```python
from build123d import *

# Parameters (mm, degrees)
CUT_EXTRUDE_1_DEPTH      = 43.811678643
PATTERN_CIRCULAR_5_COUNT = 3
EXTRUDE_1_DEPTH          = 4
SKETCH_5_R               = 14
CUT_EXTRUDE_2_DEPTH      = 45.179631373
SKETCH_6_R               = 7
CUT_EXTRUDE_3_DEPTH      = 45.17963138
SKETCH_7_W               = 30.2
SKETCH_7_H               = 16.2
CUT_EXTRUDE_4_DEPTH      = 3.35
EXTRUDE_START            = -0.2
SKETCH_8_R               = 7
EXTRUDE_2_DEPTH          = 0.2


with BuildPart() as part:
    # Sketch 1 → Revolve 1 (revolve)
    with BuildSketch(Plane.XY):
        with BuildLine():
            Line((11.135528726, 0), (28.991378029, 0))
            Line((28.991378029, 0), (28.991378029, 10.908116908))
            Line((28.991378029, 10.908116908), (27.577164466, 12.32233047))
            Line((27.577164466, 12.32233047), (26.673957337, 12.32233047))
            ThreePointArc((26.673957337, 12.32233047), (19.883391716, 4.927091635), (11.135528726, 0))
        make_face()
    revolve(axis=Axis((0, 0, 0), (0, 1, 0)))

    # Sketch 2 → Cut-Extrude 1 (cut, through all)
    with BuildSketch(Plane.XZ):
        with BuildLine():
            Line((4.04141358, 7), (4.04141358, -7))
            Line((4.04141358, -7), (34.14370091, -7))
            ThreePointArc((34.14370091, -7), (-34.85387083, 0), (34.14370091, 7))
            Line((34.14370091, 7), (28.133609793, 7))
            Line((28.133609793, 7), (4.04141358, 7))
        make_face()
    extrude(amount=-CUT_EXTRUDE_1_DEPTH, mode=Mode.SUBTRACT)

    # Sketch 3 → Cut-Revolve 3 (revolve, cut)
    with BuildSketch(Plane.XY):
        with BuildLine():
            Line((21.213203436, 8.786796564), (24.04163056, 5.95836944))
            ThreePointArc((24.04163056, 5.95836944), (21.213203436, 5.95836944), (21.213203436, 8.786796564))
        make_face()
    revolve(axis=Axis((0, 30, 0), (0.7071067811865439, -0.7071067811865512, 0)), mode=Mode.SUBTRACT)


with BuildPart() as pattern_circular_5_1:
    # Pattern Circular 5: pattern copy
    add(part.part.rotate(Axis((0, 0, 0), (0, 1, 0)), 1 * 360 / PATTERN_CIRCULAR_5_COUNT))


with BuildPart() as pattern_circular_5_2:
    # Pattern Circular 5: pattern copy
    add(part.part.rotate(Axis((0, 0, 0), (0, 1, 0)), 2 * 360 / PATTERN_CIRCULAR_5_COUNT))


with BuildPart() as part_1:
    add(part.part)

    add(pattern_circular_5_1.part)  # Extrude 1 merges Pattern Circular 5_1

    add(pattern_circular_5_2.part)  # Extrude 1 merges Pattern Circular 5_2
    # Sketch 4 → Extrude 1 (add)
    with BuildSketch(Plane.XZ):
        with BuildLine():
            Line((-20, -30), (20, -30))
            ThreePointArc((20, -30), (27.071067812, -27.071067812), (30, -20))
            Line((30, -20), (30, 20))
            ThreePointArc((30, 20), (27.071067812, 27.071067812), (20, 30))
            Line((20, 30), (-20, 30))
            ThreePointArc((-20, 30), (-27.071067812, 27.071067812), (-30, 20))
            Line((-30, 20), (-30, -20))
            ThreePointArc((-30, -20), (-27.071067812, -27.071067812), (-20, -30))
        make_face()
    extrude(amount=EXTRUDE_1_DEPTH)

    # Sketch 5 → Cut-Extrude 2 (cut, through all)
    with BuildSketch(Plane(origin=(0, 0, 0), x_dir=(1, 0, 0), z_dir=(0, 1, 0))):
        Circle(SKETCH_5_R)
    extrude(amount=CUT_EXTRUDE_2_DEPTH, mode=Mode.SUBTRACT)

    # Sketch 6 → Cut-Extrude 3 (cut, through all)
    with BuildSketch(Plane(origin=(0, 0, 0), x_dir=(1, 0, 0), z_dir=(0, 1, 0))):
        with Locations(Location((0, 0, 0), (0, 0, 180))):
            Circle(SKETCH_6_R)
    extrude(amount=-CUT_EXTRUDE_3_DEPTH, mode=Mode.SUBTRACT)

    # Sketch 7 → Cut-Extrude 4 (cut)
    with BuildSketch(Plane.XZ.offset(4)):
        with Locations((1, 0)):
            Rectangle(SKETCH_7_W, SKETCH_7_H)
    extrude(amount=-CUT_EXTRUDE_4_DEPTH, mode=Mode.SUBTRACT)

    # Sketch 8 → Extrude 2 (add)
    with BuildSketch(Plane.XZ.offset(0.65).offset(EXTRUDE_START)):
        with Locations(Location((0, 0, 0), (0, 0, 180))):
            Circle(SKETCH_8_R)
    extrude(amount=EXTRUDE_2_DEPTH)


solid = part_1.part
```
Here's how the part is built. I have some questions about the finished solid (model axes, mm). A direction names the side the tool comes from. Coordinates: 2 decimals unless noted, no trailing zeros. Order: outer loops, then holes, each group sorted by start corner. A loop starts at its lowest first (then second) coordinate and runs counter-clockwise, first axis right, second up.
1) I need wall thicknesses on line 1 (Z direction, x = 0, y = -0.1); line 2 (Z direction, x = 3.5, y = -2.5). Which ranges of each line are inside material? Lowest first, please.
2) Imagine slicing it at C-C on z = 0. List the corners of the cut face in (x, y) for me.
3) Will these pins go through, and if not, where does the flat tip stop? pin 1 (5 mm diameter, centred on x = 16.5, y = 7, fed in from -Z); pin 2 (4 mm diameter, centred on x = -1.5, z = 2, fed in from +Y); pin 3 (6 mm diameter, centred on x = 21.5, y = 7, fed in from -Z); pin 4 (5 mm diameter, centred on x = -22, z = -11, fed in from +Y).
4) We'd pull the mould along Z, two halves only. Please class faces 5 (the face through (28.1, 11.8, 0.1)), 6 (the face through (-17.07, 4.71, 15.57)), 7 (the face through (27, 12.322, 0)), 8 (the face through (-14.15, 11.78, 24.3)): +Z half, -Z half, draft (parallel to the pull), parting line (faces both ways), or undercut.
5) Imagine slicing it at A-A on x = 8. List the corners of the cut face in (y, z) for me, and give its area (3 significant figures).
6) Which directions (+Z, -Z, +X, -X, +Y, -Y) give clear straight access to the entire face, cutting with the end or side of a thin tool? Please do faces 1 (the face through (1, -2, 8.1)), 2 (the face through (22, 5, 7)), 3 (the face through (28.99, 5.53, 0.1)), 4 (the face through (0, -0.45, 0)).
7) Imagine slicing it at D-D on x = -25. List the corners of the cut face in (y, z) for me.
8) Imagine slicing it at B-B on y = -2. List the corners of the cut face in (x, z) for me, and give its area (3 significant figures).
Response values:
1. line 1: z = -30 to -7, 7 to 30
1. line 2: z = -30 to -8.1, 8.1 to 30
2. outline: (-30, -4) - (-14.1, -4) - (-14.1, -0.65) - (16.1, -0.65) - (16.1, -4) - (30, -4) - (30, 0) - (28.99, 0) - (28.99, 10.91) - (27.58, 12.32) - (26.67, 12.32) arc R32 cw to (24, 8.83) arc R2 cw (long way) to (21.17, 6) arc R32 cw to (14, 1.23) - (14, 0) - (7, 0) - (7, -0.45) - (-7, -0.45) - (-7, 0) - (-30, 0) - close
3. pin 1: passes through
3. pin 2: stops at y = -0.45
3. pin 3: stops at z = -7
3. pin 4: stops at y = 0
4. face 5: parting line
4. face 6: undercut
4. face 7: draft
4. face 8: +Z half
5. outline: (-4, -30) - (0, -30) - (0, 30) - (-4, 30) - (-4, 8.1) - (-0.65, 8.1) - (-0.65, -8.1) - (-4, -8.1) - close
5. area: 186 mm2
6. face 1: -Y
6. face 2: +Z, +X, +Y
6. face 3: +X, +Y
6. face 4: +Y
7. outline: (-4, -28.66) - (0, -28.66) - (0, 28.66) - (-4, 28.66) - close
8. outline: (-30, -20) arc R10 ccw to (-20, -30) - (20, -30) arc R10 ccw to (30, -20) - (30, 20) arc R10 ccw to (20, 30) - (-20, 30) arc R10 ccw to (-30, 20) - close; hole (-14.1, -8.1) - (16.1, -8.1) - (16.1, 8.1) - (-14.1, 8.1) - close
8. area: 3,020 mm2
